from build123d import *

# Parameters (mm, degrees)
F0_W     = 38.1
F0_H     = 31.75
F1_DEPTH = 25.4
F2_W     = 25.4
F2_H     = 25.4
F3_DEPTH = 19.05
F5_DEPTH = 25.4


with BuildPart() as f1:
    # F0 (on Top) → F1 (new body)
    with BuildSketch(Plane.XY):
        with Locations((19.05, 15.875)):
            Rectangle(F0_W, F0_H)
    extrude(amount=F1_DEPTH)

    # F2 (on face) → F3 (cut)
    with BuildSketch(Plane.XY.offset(25.4)):
        with Locations((25.4, 12.7)):
            Rectangle(F2_W, F2_H)
    extrude(amount=-F3_DEPTH, mode=Mode.SUBTRACT)

    # F4 (on Top) → F5 (cut)
    with BuildSketch(Plane.XY):
        Polygon((38.1, 12.7), (0, 0), (38.1, 0), align=None)
    extrude(amount=F5_DEPTH, mode=Mode.SUBTRACT)


solid = f1.part
Geometry: final body of the model. Coordinates: model frame, mm. A direction names the side the tool comes from. Coordinates: 2 decimals unless noted, no trailing zeros. Loops run counter-clockwise (first coordinate to the right, second up) from the corner with the lowest first, then second, coordinate; pieces in that order, holes last. Notation, with made-up numbers: M 83,72 L 110,72 A19 cw 110,91 Z; hole C 30.25,71 d11. An arc over 180 degrees is marked long. One line per item, written item: value. Start each with the question number.
1) Material intervals for L1, parallel to X at y = 23.5, z = 24; L2, parallel to Z at x = 35, y = 21; L3, parallel to Y at x = 37, z = 16.25, sorted ascending. Write a range as from..to.
2) Cut plane D-D (x = 7). Return loops of the section in (y, z), then the cut area to 3 significant figures.
3) Cut plane A-A (y = 11). Return loops of the section in (x, z).
4) Cut plane B-B (x = 18). Return loops of the section in (y, z), then the cut area to 3 significant figures.
5) Pin query (flat end, axial travel): P1, Ø1, axis at x = 33.5, z = 10.5, coming from the -Y side; P2, Ø3, axis at x = 29.5, y = 13.5, coming from the +Z side; P3, Ø3, axis at y = 14, z = 20, coming from the +X side. Return the tip coordinate at first contact, or that it passes through.
6) Reachability of faces 1 (the flat face through (10.85, 3.617, 9.7)), 2 (the flat face through (25, 17, 6.35)) from +Z, -Z, +X, -X, +Y, -Y: full face, straight path, thin tool, end or side. Return the list, or none.
7) Cut plane C-C (z = 3.25). Return loops of the section in (x, y), then the cut area to 3 significant figures.
Evaluation:
1. L1: 0..12.7
1. L2: 0..6.35
1. L3: 25.4..31.75
2. outline: M 2.33,0 L 31.75,0 L 31.75,25.4 L 2.33,25.4 Z
2. area: 747 mm^2
3. outline: M 0,0 L 33,0 L 33,6.35 L 12.7,6.35 L 12.7,25.4 L 0,25.4 Z
4. outline: M 6,0 L 31.75,0 L 31.75,25.4 L 25.4,25.4 L 25.4,6.35 L 6,6.35 Z
4. area: 284 mm^2
5. P1: y = 25.4
5. P2: z = 6.35
5. P3: x = 12.7
6. face 1: +Z, -Z, +X, -Y
6. face 2: +Z, +X, -Y
7. outline: M 0,0 L 38.1,12.7 L 38.1,31.75 L 0,31.75 Z
7. area: 968 mm^2
